```python
from build123d import *

# Parameters (mm, degrees)
SKETCH1_W               = 15
SKETCH1_H               = 20
BOSS_EXTRUDE1_DEPTH     = 25
CUT_EXTRUDE1_DEPTH      = 31.822070015
CUT_EXTRUDE1_DEPTH_BACK = 31.822070015
SKETCH2_R               = 7.5
M6_TAPPED_HOLE1_D       = 5


with BuildPart() as part:
    # Sketch1 → Boss-Extrude1 (new, symmetric)
    with BuildSketch(Plane(origin=(0, 0, 0), x_dir=(0, 0, -1), z_dir=(1, 0, 0))):
        Rectangle(SKETCH1_W, SKETCH1_H)
    extrude(amount=BOSS_EXTRUDE1_DEPTH, both=True)

    # Sketch2 → Cut-Extrude1 (cut, two sides: drawn at the far end of the back side and taken through both)
    with BuildSketch(Plane.XY.offset(7.5).offset(-CUT_EXTRUDE1_DEPTH_BACK)):
        with Locations((15, 0)):
            Circle(SKETCH2_R)
    extrude(amount=CUT_EXTRUDE1_DEPTH + CUT_EXTRUDE1_DEPTH_BACK, mode=Mode.SUBTRACT)

    # M6 Tapped Hole1 (through all)
    with Locations(Plane.XY.offset(7.5)):
        with Locations((0, 0), (-20, 0)):
            Hole(M6_TAPPED_HOLE1_D / 2)


solid = part.part
```
Work out the finished part from the listing and answer in its coordinate system (mm). Coordinates: 2 decimals unless noted, no trailing zeros. Loops run counter-clockwise (first coordinate to the right, second up) from the corner with the lowest first, then second, coordinate; pieces in that order, holes last. Notation, with made-up numbers: (25, -20) - (49, -20) arc R18 ccw to (49, -12) - close; hole circle Ø1 at (44, 25). An arc over 180 degrees is marked (long way). Use a Markdown table: item, result.
Item 1: Consider probe 1 along Y at (x, z) = (15, 3.5); probe 2 along X at (y, z) = (2, -6); probe 3 along Y at (x, z) = (0, 1.25). Determine where each line is inside the solid, lowest interval first. Write a range as from..to.
Evaluation:
| item | result |
|---|---|
| probe 1 | y = -10..-7.5, 7.5..10 |
| probe 2 | x = -25..-21.5, -18.5..-1.5, 1.5..7.77, 22.23..25 |
| probe 3 | y = -10..-2.5, 2.5..10 |
Item 2: Find section D-D, the plane z = -2.25. Determine the outline of the cut face in (x, y), and give its area (3 significant figures).
Evaluation:
| item | result |
|---|---|
| outline | (-25, -10) - (25, -10) - (25, 10) - (-25, 10) - close; hole circle Ø5 at (-20, 0); hole circle Ø5 at (0, 0); hole circle Ø15 at (15, 0) |
| area | 784 mm2 |
Item 3: The mould has two halves that part along X. Classify faces 1 (the flat face through (-25, 0, 0)), 2 (the cylindrical face through (7.507, 0.33, -0.105)), 3 (the flat face through (25, 0, 0)), 4 (the cylindrical face through (0.54, -2.44, -0.11)): +X half, -X half, draft (parallel to the pull), parting line (faces both ways), or undercut.
Evaluation:
| item | result |
|---|---|
| face 1 | -X half |
| face 2 | undercut |
| face 3 | +X half |
| face 4 | undercut |
Item 4: Find section A-A, the plane y = 0. Determine the outline of the cut face in (x, z), and give its area (3 significant figures).
Evaluation:
| item | result |
|---|---|
| outline | (-25, -7.5) - (-22.5, -7.5) - (-22.5, 7.5) - (-25, 7.5) - close; (-17.5, -7.5) - (-2.5, -7.5) - (-2.5, 7.5) - (-17.5, 7.5) - close; (2.5, -7.5) - (7.5, -7.5) - (7.5, 7.5) - (2.5, 7.5) - close; (22.5, -7.5) - (25, -7.5) - (25, 7.5) - (22.5, 7.5) - close |
| area | 375 mm2 |
Item 5: Given pin 1 Ø1 at (x, y) = (10, 2.5) entering from +Z, flat-ended and moving along its own axis, determine where the tip first touches the part or whether it passes through.
Evaluation:
| item | result |
|---|---|
| pin 1 | passes through |
Item 6: Find section C-C, the plane y = 6.25. Determine the outline of the cut face in (x, z).
Evaluation:
| item | result |
|---|---|
| outline | (-25, -7.5) - (10.85, -7.5) - (10.85, 7.5) - (-25, 7.5) - close; (19.15, -7.5) - (25, -7.5) - (25, 7.5) - (19.15, 7.5) - close |
Item 7: Find section B-B, the plane x = 15. Determine the outline of the cut face in (y, z), and give its area (3 significant figures).
Evaluation:
| item | result |
|---|---|
| outline | (-10, -7.5) - (-7.5, -7.5) - (-7.5, 7.5) - (-10, 7.5) - close; (7.5, -7.5) - (10, -7.5) - (10, 7.5) - (7.5, 7.5) - close |
| area | 75.0 mm2 |
